Autodesk Inventor part; units mm, degrees
ref_plane "YZ Plane" through (0, 0, 0) normal (1, 0, 0) x (0, 1, 0)
ref_plane "XZ Plane" through (0, 0, 0) normal (0, 1, 0) x (-1, 0, 0)
ref_plane "XY Plane" through (0, 0, 0) normal (0, 0, 1) x (1, 0, 0)
sketch "Sketch1" plane through (0, 0, 0) normal (0, 0, 1) x (1, 0, 0)
  line L0 (0, 0) -> (0, 19.4488) construction
  line L1 (0, 0) -> (15.8946, 0) construction
  line L2 (1.61, 5) -> (6.7, 5)
  line L3 (6.7, 5) -> (6.7, 0)
  line L4 (6.7, 0) -> (12.5, 0)
  line L5 (12.5, 0) -> (12.5, 12.791)
  line L6 (1.0049, 10.15) -> (0.7849, 10.15) construction
  line L7 (1.6103, 4.761) -> (2.6467, 18.8742) construction
  line L8 (0.4645, 3.15) -> (0.2, 3.15) construction
  line L9 (0, 2.7) -> (1.1563, 2.7) construction
  line L10 (12.5, 12.791) -> (2.2, 12.791)
  line L11 (2.2, 12.791) -> (1.61, 5)
  point P0 (9.6, 0)
  dimension "d1" = 12.5
  dimension "d2" = 6.7
  dimension "d7" = 5
  dimension "d53" = 0.22
  dimension "d55" = 0.2
  dimension "d58" = 2.3
  dimension "d62" = 1.61
  dimension "d63" = 2.2
  dimension "d64" = 12.791
revolve "Revolution1" add sketch "Sketch1" angle 360 about axis through (0, 0, 0) along (0, 1, 0)
chamfer "Chamfer2" distance 1 angle 45 2 edges at (-12.5, 0, 0) (-12.5, 12.791, 0)
sketch "Sketch7" plane through (0, 12.791, 0) normal (0, 1, 0) x (1, 0, 0)
  circle A0 centre (0, 0) radius 10.5 construction
  line L0 (0, 0) -> (23.4924, 0) construction
  line L1 (0, 0) -> (0, 17.9898) construction
  line L2 (0, 0) -> (-15.6301, 15.6301) construction
  circle A1 centre (-7.4246, 7.4246) radius 0.75
  point P0 (12.4999, 0)
  dimension "d84" = 21
  dimension "d85" = 45
  dimension "d86" = 1.5
extrude "Extrusion6" cut sketch "Sketch7" against normal blind 1.7
sketch "Sketch8" plane through (0, 12.791, 0) normal (0, 1, 0) x (1, 0, 0)
  circle A0 centre (0, 0) radius 12.5 construction
  line L0 (0, 0) -> (0, 17.9558) construction
  circle A1 centre (0, 12.5) radius 2.5
  dimension "d89" = 25
  dimension "d90" = 5
extrude "Extrusion7" cut sketch "Sketch8" against normal blind 12.791
pattern_circular "Circular Pattern4" count 4 over 360 about axis through (0, 8.8955, 0) along (0, -1, 0) of "Extrusion6", "Extrusion7"
sketch "Sketch9" plane through (0, 12.791, -12.5) normal (0, 1, 0) x (1, 0, 0)
  circle A0 centre (0, -12.5) radius 6
  circle A1 centre (0, -12.5) radius 2.5
  dimension "d96" = 12
  dimension "d97" = 5
extrude "Extrusion8" add sketch "Sketch9" along normal blind 4.9
chamfer "Chamfer7" distance 1 angle 45 1 edges at (-6, 17.691, 0)
chamfer "Chamfer8" distance 0.5 angle 45 1 edges at (-2.5, 17.691, 0)
sketch "Sketch10" plane through (0, 0, -12.5) normal (0, -1, 0) x (1, 0, 0)
  circle A0 centre (0, 12.5) radius 10.5 construction
  line L0 (0, 12.5) -> (14.2322, 12.5) construction
  line L1 (0, 12.5) -> (13.4469, 25.9469) construction
  circle A1 centre (7.4246, 19.9246) radius 0.75
  dimension "d106" = 21
  dimension "d107" = 45
  dimension "d108" = 1.5
extrude "Extrusion9" add sketch "Sketch10" along normal blind 1.5
chamfer "Chamfer9" distance 0.35 angle 45 1 edges at (6.6746, -1.5, 7.4246)
pattern_circular "Circular Pattern5" count 4 over 360 about axis through (0, 2.5, 0) along (0, -1, 0) of "Extrusion9", "Chamfer9"
equation "\"cutpipette_length\" = 5.7"
properties part number "cpd_lowrcf_1.3_p2_20230620"
Check sheet for the modelled part. Datum: model origin and axes. Units: mm. A direction names the side the tool comes from. Give positions to 0.01 mm unless a question says otherwise; leave off trailing zeros. Order: outer loops, then holes, each group sorted by start corner. A loop starts at its lowest first (then second) coordinate and runs counter-clockwise, first axis right, second up. Notation, with made-up numbers: (-1, 17.25) - (25, 17.25) arc R23 ccw to (25, 27.25) - close; hole circle Ø8 at (84.5, 3.25). An arc over 180 degrees is marked (long way). Answer as CSV lines item,"result".
1. Section check B-B (y = 3.5). Record the boundary of the cut face in (x, z), then the cut area to 3 significant figures.
Result sheet:
outline,"(-12.25, -2.49) arc R12.5 ccw to (-2.49, -12.25) arc R2.5 cw to (2.49, -12.25) arc R12.5 ccw to (12.25, -2.49) arc R2.5 cw to (12.25, 2.49) arc R12.5 ccw to (2.49, 12.25) arc R2.5 cw to (-2.49, 12.25) arc R12.5 ccw to (-12.25, 2.49) arc R2.5 cw to start; hole circle Ø13.4 at (0, 0)"
area,"312 mm²"
2. Section check C-C (z = 0). Record the boundary of the cut face in (x, y).
Result sheet:
outline,"(-10, 0) - (-6.7, 0) - (-6.7, 5) - (-1.61, 5) - (-2.2, 12.79) - (-2.5, 12.79) - (-2.5, 17.19) - (-3, 17.69) - (-5, 17.69) - (-6, 16.69) - (-6, 12.79) - (-10, 12.79) - close; (1.61, 5) - (6.7, 5) - (6.7, 0) - (10, 0) - (10, 12.79) - (6, 12.79) - (6, 16.69) - (5, 17.69) - (3, 17.69) - (2.5, 17.19) - (2.5, 12.79) - (2.2, 12.79) - close"
3. Section check A-A (x = 0). Record the boundary of the cut face in (y, z), then the cut area to 3 significant figures.
Result sheet:
outline,"(0, -10) - (12.79, -10) - (12.79, -6) - (16.69, -6) - (17.69, -5) - (17.69, -3) - (17.19, -2.5) - (12.79, -2.5) - (12.79, -2.2) - (5, -1.61) - (5, -6.7) - (0, -6.7) - close; (0, 6.7) - (5, 6.7) - (5, 1.61) - (12.79, 2.2) - (12.79, 2.5) - (17.19, 2.5) - (17.69, 3) - (17.69, 5) - (16.69, 6) - (12.79, 6) - (12.79, 10) - (0, 10) - close"
area,"192 mm²"
4. Tool access check on faces 1 (the face through (-8.766, 6.471, -8.911)), 2 (the face through (7.4, 11.091, 7.4)), 3 (the face through (7.33, -0.57, 6.68)). Record the directions out of +Z, -Z, +X, -X, +Y, -Y that give a thin tool (end or side, any length) a straight path to the whole face; none if there is none.
Result sheet:
face 1,"-Z, -X, +Y, -Y"
face 2,"+Y"
face 3,"-Y"
5. Go/stop test with flat-tipped pins: P1, Ø0.8, axis at x = -7.5, z = 7.5, coming from the +Y side; P2, Ø10, axis at x = 6, y = 10.5, coming from the +Z side; P3, Ø1.7, axis at x = -7.42, z = -7.42, coming from the +Y side; P4, Ø7, axis at x = -3.5, z = 3, coming from the -Y side. Record where each tip stops, or that it passes through.
Result sheet:
P1,"y = 11.09"
P2,"z = 12.25"
P3,"y = 12.79"
P4,"y = 0"
6. Mould release check, pull along Z, two halves, no side actions. Record for faces 4 (the face through (-8.186, 0.174, -8.323)), 5 (the face through (6.68, -0.57, -7.33)), 6 (the face through (-7.4, -1.5, 7.4)): released by +Z, released by -Z, zero draft, split by the parting line, or undercut.
Result sheet:
face 4,"released by -Z"
face 5,"undercut"
face 6,"zero draft"
7. Scan lines: probe 1 along X at (y, z) = (14.2, 0); probe 2 along Y at (x, z) = (-5, -8.75). Record each from-to range of solid material in increasing order. Write a range as from..to.
Result sheet:
probe 1,"-6..-2.5, 2.5..6"
probe 2,"0..12.79"
8. Section check D-D (y = 7.25). Record the boundary of the cut face in (x, z), then the cut area to 3 significant figures.
Result sheet:
outline,"(-12.25, -2.49) arc R12.5 ccw to (-2.49, -12.25) arc R2.5 cw to (2.49, -12.25) arc R12.5 ccw to (12.25, -2.49) arc R2.5 cw to (12.25, 2.49) arc R12.5 ccw to (2.49, 12.25) arc R2.5 cw to (-2.49, 12.25) arc R12.5 ccw to (-12.25, 2.49) arc R2.5 cw to start; hole circle Ø3.56 at (0, 0)"
area,"443 mm²"
